```python
from build123d import *

# Parameters (mm, degrees)
SKETCH1_W           = 231.05
SKETCH1_H           = 88.9
SKETCH1_R           = 15
SKETCH1_R_2         = 2.5
SKETCH1_R_3         = 3
SKETCH1_R_4         = 4
BOSS_EXTRUDE1_DEPTH = 3.6


with BuildPart() as part:
    # Sketch1 → Boss-Extrude1 (new body)
    with BuildSketch(Plane(origin=(0, 0, 0), x_dir=(1, 0, 0), z_dir=(0, 1, 0))):
        with Locations((-115.525, 0)):
            Rectangle(SKETCH1_W, SKETCH1_H)
        with Locations((-183.9, 0)):
            Circle(SKETCH1_R, mode=Mode.SUBTRACT)
        with Locations((-47.15, 0)):
            Circle(SKETCH1_R, mode=Mode.SUBTRACT)
        with Locations((-63.15, -16)):
            Circle(SKETCH1_R_2, mode=Mode.SUBTRACT)
        with Locations((-31.15, -16)):
            Circle(SKETCH1_R_2, mode=Mode.SUBTRACT)
        with Locations((-31.15, 16)):
            Circle(SKETCH1_R_2, mode=Mode.SUBTRACT)
        with Locations((-63.15, 16)):
            Circle(SKETCH1_R_2, mode=Mode.SUBTRACT)
        with Locations((-167.9, 16)):
            Circle(SKETCH1_R_2, mode=Mode.SUBTRACT)
        with Locations((-199.9, 16)):
            Circle(SKETCH1_R_2, mode=Mode.SUBTRACT)
        with Locations((-199.9, -16)):
            Circle(SKETCH1_R_2, mode=Mode.SUBTRACT)
        with Locations((-167.9, -16)):
            Circle(SKETCH1_R_2, mode=Mode.SUBTRACT)
        with Locations((-139.15, -2.858987694)):
            Circle(SKETCH1_R_3, mode=Mode.SUBTRACT)
        with Locations((-91.9, 2.858987694)):
            Circle(SKETCH1_R_3, mode=Mode.SUBTRACT)
        with Locations((-218.35, 0)):
            Circle(SKETCH1_R_4, mode=Mode.SUBTRACT)
        with Locations((-12.7, 0)):
            Circle(SKETCH1_R_4, mode=Mode.SUBTRACT)
    extrude(amount=-BOSS_EXTRUDE1_DEPTH)


solid = part.part
```
Input: part model. Units: mm. Frame: model coordinates. Give positions to 0.01 mm unless a question says otherwise; leave off trailing zeros. Order: outer loops, then holes, each group sorted by start corner. A loop starts at its lowest first (then second) coordinate and runs counter-clockwise, first axis right, second up. Notation, with made-up numbers: M -5.5,-18 L 31.5,-18 A33 cw 31.5,11 Z; hole C -37.5,18.5 d2. An arc over 180 degrees is marked long. One line per question, with ' | ' between items.
1) Ray query, L1, parallel to Z at x = -199.9, y = -2.8; L2, parallel to X at y = -1.5, z = 16; L3, parallel to Z at x = -91.9, y = -1.1. Return the intervals inside material, ascending.
Filled in:
L1: z = -44.45 to -18.5, -13.5 to 13.5, 18.5 to 44.45 | L2: x = -231.05 to -202.4, -197.4 to -170.4, -165.4 to -65.65, -60.65 to -33.65, -28.65 to 0 | L3: z = -44.45 to -5.86, 0.14 to 44.45
2) Section A-A on x = -91.9. Output: boundary loops of the cut face in (y, z).
Filled in:
outline: M -3.6,-44.45 L 0,-44.45 L 0,-5.86 L -3.6,-5.86 Z; M -3.6,0.14 L 0,0.14 L 0,44.45 L -3.6,44.45 Z
3) Section B-B on x = -183.9. Output: boundary loops of the cut face in (y, z).
Filled in:
outline: M -3.6,-44.45 L 0,-44.45 L 0,-15 L -3.6,-15 Z; M -3.6,15 L 0,15 L 0,44.45 L -3.6,44.45 Z
4) Draft query along X for faces 1 (the face through (-16.696, -1.775, -0.176)), 2 (the face through (-117, 0, -1)). Return one class per face: pulls with the +X half, pulls with the -X half, needs draft (parallel to the pull), parting line crosses it, or undercut.
Filled in:
face 1: undercut | face 2: needs draft
